Part model, mm, in its own coordinate system. Give positions to 0.01 mm unless a question says otherwise; leave off trailing zeros. Order: outer loops, then holes, each group sorted by start corner. A loop starts at its lowest first (then second) coordinate and runs counter-clockwise, first axis right, second up. Notation, with made-up numbers: (51, 56.5) - (89, 56.5) arc R16 ccw to (89, 71.5) - close; hole circle Ø6 at (-38, 1). An arc over 180 degrees is marked (long way). One line per item, written item: value.
```python
from build123d import *

# Parameters (mm, degrees)
SKETCH1_W                                         = 76.2
SKETCH1_H                                         = 12.7
BOSS_EXTRUDE2_DEPTH                               = 4.7625
F_4_CLEARANCE_HOLE1_D                             = 3.2639
CSK_FOR_4_FLAT_HEAD_SOCKET_CAP_SCREW2_D           = 3.2639
CSK_FOR_4_FLAT_HEAD_SOCKET_CAP_SCREW2_CSINK_D     = 6.477
CSK_FOR_4_FLAT_HEAD_SOCKET_CAP_SCREW2_CSINK_ANGLE = 82
CHAMFER1_SIZE                                     = 0.508


with BuildPart() as part:
    # Sketch1 → Boss-Extrude2 (new body)
    with BuildSketch(Plane(origin=(0, 0, 0), x_dir=(1, 0, 0), z_dir=(0, 1, 0))):
        with Locations((-31.75, 0)):
            Rectangle(SKETCH1_W, SKETCH1_H)
    extrude(amount=BOSS_EXTRUDE2_DEPTH)

    # #4 Clearance Hole1 (through all)
    with Locations(Plane(origin=(0, 4.7625, 0), x_dir=(1, 0, 0), z_dir=(0, 1, 0))):
        with Locations((-63.5, 0)):
            Hole(F_4_CLEARANCE_HOLE1_D / 2)

    # CSK for #4 Flat Head Socket Cap Screw2 (through all)
    with Locations(Plane(origin=(0, 0, 0), x_dir=(-1, 0, 0), z_dir=(0, -1, 0))):
        with Locations((0, 0)):
            CounterSinkHole(CSK_FOR_4_FLAT_HEAD_SOCKET_CAP_SCREW2_D / 2, CSK_FOR_4_FLAT_HEAD_SOCKET_CAP_SCREW2_CSINK_D / 2, counter_sink_angle=CSK_FOR_4_FLAT_HEAD_SOCKET_CAP_SCREW2_CSINK_ANGLE)

    # Chamfer1
    chamfer1_edges = [part.edges().sort_by_distance(p)[0] for p in [
        (-69.85, 2.38125, 6.35),
        (-69.85, 2.38125, -6.35),
        (6.35, 2.38125, -6.35),
        (6.35, 2.38125, 6.35),
        (6.35, 4.7625, 0),
        (-69.85, 4.7625, 0),
        (-69.85, 0, 0),
        (6.35, 0, 0),
    ]]
    chamfer(chamfer1_edges, length=CHAMFER1_SIZE)


solid = part.part
```
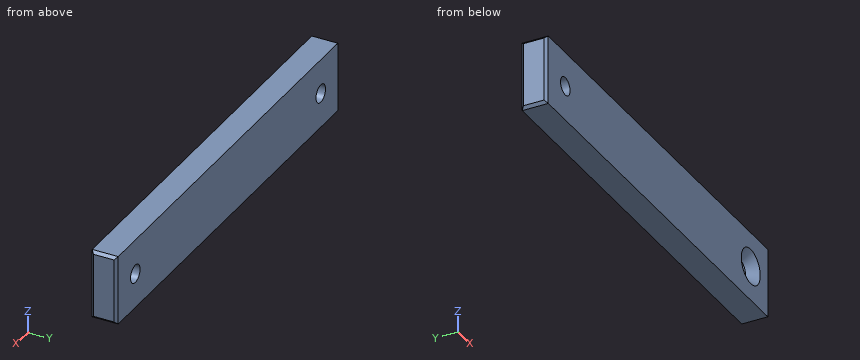
1) Pin check, flat tip, straight feed: pin 1 (2 mm diameter, centred on x = 0, z = 0, fed in from -Y). Stop position of the tip, or through.
Outcome:
pin 1: passes through
2) Cut at A-A, the plane z = 0. Give the cut face in (x, y), then the cut area to 3 significant figures.
Outcome:
outline: (-69.85, 0.51) - (-69.34, 0) - (-65.13, 0) - (-65.13, 4.76) - (-69.34, 4.76) - (-69.85, 4.25) - close; (-61.87, 0) - (-3.24, 0) - (-1.63, 1.85) - (-1.63, 4.76) - (-61.87, 4.76) - close; (1.63, 1.85) - (3.24, 0) - (5.84, 0) - (6.35, 0.51) - (6.35, 4.25) - (5.84, 4.76) - (1.63, 4.76) - close
area: 328 mm^2
3) Cut at C-C, the plane y = 3.2. Give the cut face in (x, z), then the cut area to 3 significant figures.
Outcome:
outline: (-69.85, -5.84) - (-69.34, -6.35) - (5.84, -6.35) - (6.35, -5.84) - (6.35, 5.84) - (5.84, 6.35) - (-69.34, 6.35) - (-69.85, 5.84) - close; hole circle Ø3.26 at (-63.5, 0); hole circle Ø3.26 at (0, 0)
area: 950 mm^2
4) Cut at B-B, the plane x = 0. Give the cut face in (y, z), then the cut area to 3 significant figures.
Outcome:
outline: (0, -6.35) - (4.76, -6.35) - (4.76, -1.63) - (1.85, -1.63) - (0, -3.24) - close; (0, 3.24) - (1.85, 1.63) - (4.76, 1.63) - (4.76, 6.35) - (0, 6.35) - close
area: 42.0 mm^2
5) Cut at D-D, the plane x = -63.5. Give the cut face in (y, z), then the cut area to 3 significant figures.
Outcome:
outline: (0, -6.35) - (4.76, -6.35) - (4.76, -1.63) - (0, -1.63) - close; (0, 1.63) - (4.76, 1.63) - (4.76, 6.35) - (0, 6.35) - close
area: 44.9 mm^2
6) Drill centre lines: line 1 along Z through (x, y) = (-63.5, 2.05); line 2 along X through (y, z) = (1.2, 0.5); line 3 along Z through (x, y) = (-65, 0.35). Where is each one in solid material? Low to high. Write a range as from..to.
Outcome:
line 1: z = -6.35..-1.63, 1.63..6.35
line 2: x = -69.85..-65.05, -61.95..-2.14, 2.14..6.35
line 3: z = -6.35..-0.64, 0.64..6.35
